Geometry: final body of the model. Coordinates: model frame, mm. Face numbers are marked on the shaded views. A direction names the side the tool comes from. Give positions to 0.01 mm unless a question says otherwise; leave off trailing zeros. Loops run counter-clockwise (first coordinate to the right, second up) from the corner with the lowest first, then second, coordinate; pieces in that order, holes last. Notation, with made-up numbers: (-19, 82) - (14, 82) arc R23 ccw to (14, 96) - close; hole circle Ø7 at (77.25, 1.25). An arc over 180 degrees is marked (long way). Use CSV: the item, a comma, the result in double quotes. Start each with the question number.
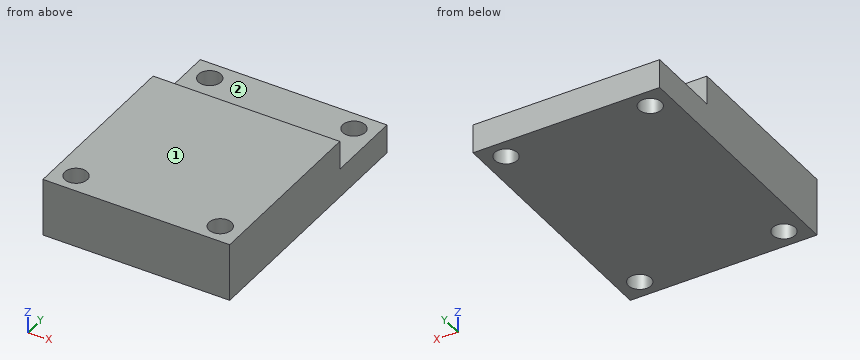
```python
from build123d import *

# Parameters (mm, degrees)
SKETCH_1_W          = 29
SKETCH_1_H          = 40
SKETCH_1_R          = 1.75
EXTRUDE_1_DEPTH     = 9
SKETCH_3_W          = 29
SKETCH_3_H          = 12
CUT_EXTRUDE_2_DEPTH = 5


with BuildPart() as part:
    # 스케치1 → 보스-돌출1 (new body)
    with BuildSketch(Plane.XY):
        Rectangle(SKETCH_1_W, SKETCH_1_H)
        with Locations((11.199423754, 17)):
            Circle(SKETCH_1_R, mode=Mode.SUBTRACT)
        with Locations((-11.199423754, 17)):
            Circle(SKETCH_1_R, mode=Mode.SUBTRACT)
        with Locations(Location((11.199423754, -17, 0), (0, 0, 180))):
            Circle(SKETCH_1_R, mode=Mode.SUBTRACT)
        with Locations(Location((-11.199423754, -17, 0), (0, 0, 180))):
            Circle(SKETCH_1_R, mode=Mode.SUBTRACT)
    extrude(amount=EXTRUDE_1_DEPTH)

    # 스케치3 → 컷-돌출2 (cut)
    with BuildSketch(Plane(origin=(0, 0, 4.5), x_dir=(-1, 0, 0), z_dir=(0, 0, -1))):
        with Locations((0, 14)):
            Rectangle(SKETCH_3_W, SKETCH_3_H)
    extrude(amount=-CUT_EXTRUDE_2_DEPTH, mode=Mode.SUBTRACT)


solid = part.part
```
Item 1: Section B-B (z = 3.25). Output: boundary loops of the cut face in (x, y), plus the area to 3 significant figures.
Item 2: Section D-D (y = -16). Output: boundary loops of the cut face in (x, z).
Item 3: Section C-C (x = -3.5). Output: boundary loops of the cut face in (y, z), plus the area to 3 significant figures.
Item 4: Pin query (flat end, axial travel): pin 1 Ø2 at (x, z) = (-1.5, 6.5) entering from +Y. Return the tip coordinate at first contact, or that it passes through.
Item 5: Reachability of the marked faces 1 and 2 from +Z, -Z, +X, -X, +Y, -Y: full face, straight path, thin tool, end or side. Return the list, or none.
Item 6: Ray query, probe 1 along X at (y, z) = (-17, 7); probe 2 along Y at (x, z) = (-1.25, 8.5); probe 3 along Z at (x, y) = (-2.5, 18). Return the intervals inside material, ascending.
Item 7: Section A-A (y = 17). Output: boundary loops of the cut face in (x, z).
Outcome:
1,outline,"(-14.5, -20) - (14.5, -20) - (14.5, 20) - (-14.5, 20) - close; hole circle Ø3.5 at (-11.2, -17); hole circle Ø3.5 at (-11.2, 17); hole circle Ø3.5 at (11.2, -17); hole circle Ø3.5 at (11.2, 17)"
1,area,"1,120 mm2"
2,outline,"(-14.5, 0) - (-12.64, 0) - (-12.64, 9) - (-14.5, 9) - close; (-9.76, 0) - (9.76, 0) - (9.76, 9) - (-9.76, 9) - close; (12.64, 0) - (14.5, 0) - (14.5, 9) - (12.64, 9) - close"
3,outline,"(-20, 0) - (20, 0) - (20, 4.5) - (8, 4.5) - (8, 9) - (-20, 9) - close"
3,area,"306 mm2"
4,pin 1,"stops at y = 8"
5,face 1,"+Z, +X, -X, +Y, -Y"
5,face 2,"+Z, +X, -X, +Y"
6,probe 1,"x = -14.5 to -12.95, -9.45 to 9.45, 12.95 to 14.5"
6,probe 2,"y = -20 to 8"
6,probe 3,"z = 0 to 4.5"
7,outline,"(-14.5, 0) - (-12.95, 0) - (-12.95, 4.5) - (-14.5, 4.5) - close; (-9.45, 0) - (9.45, 0) - (9.45, 4.5) - (-9.45, 4.5) - close; (12.95, 0) - (14.5, 0) - (14.5, 4.5) - (12.95, 4.5) - close"
